Part model, mm, in its own coordinate system. Coordinates: 2 decimals unless noted, no trailing zeros. Loops run counter-clockwise (first coordinate to the right, second up) from the corner with the lowest first, then second, coordinate; pieces in that order, holes last. Notation, with made-up numbers: (84.25, 6) - (102.25, 6) arc R17 cw to (102.25, 29) - close; hole circle Ø5 at (88, 44.25). An arc over 180 degrees is marked (long way). Answer as CSV lines item,"result".
from build123d import *

# Parameters (mm, degrees)
F1_DEPTH = 1622.425
F3_DEPTH = 38.1
F5_DEPTH = 25.4


with BuildPart() as f1:
    # F0 (on Front) → F1 (new body)
    with BuildSketch(Plane.XZ):
        with BuildLine():
            Line((-10.2273916114, -12.0247762322), (8.8226083886, -12.0247762322))
            ThreePointArc((8.8226083886, -12.0247762322), (11.0676724189, -11.0948402625), (11.9976083886, -8.8497762322))
            Line((11.9976083886, -8.8497762322), (11.9976083886, 10.2002237678))
            ThreePointArc((11.9976083886, 10.2002237678), (11.0676724189, 12.445287798), (8.8226083886, 13.3752237678))
            Line((8.8226083886, 13.3752237678), (-10.2273916114, 13.3752237678))
            ThreePointArc((-10.2273916114, 13.3752237678), (-12.4724556417, 12.445287798), (-13.4023916114, 10.2002237678))
            Line((-13.4023916114, 10.2002237678), (-13.4023916114, -8.8497762322))
            ThreePointArc((-13.4023916114, -8.8497762322), (-12.4724556417, -11.0948402625), (-10.2273916114, -12.0247762322))
        make_face()
        with BuildLine():
            ThreePointArc((8.8226083886, -5.6747762322), (7.8926724189, -7.9198402625), (5.6476083886, -8.8497762322))
            Line((5.6476083886, -8.8497762322), (-7.0523916114, -8.8497762322))
            ThreePointArc((-7.0523916114, -8.8497762322), (-9.2974556417, -7.9198402625), (-10.2273916114, -5.6747762322))
            Line((-10.2273916114, -5.6747762322), (-10.2273916114, 7.0252237678))
            ThreePointArc((-10.2273916114, 7.0252237678), (-9.2974556417, 9.270287798), (-7.0523916114, 10.2002237678))
            Line((-7.0523916114, 10.2002237678), (5.6476083886, 10.2002237678))
            ThreePointArc((5.6476083886, 10.2002237678), (7.8926724189, 9.270287798), (8.8226083886, 7.0252237678))
            Line((8.8226083886, 7.0252237678), (8.8226083886, -5.6747762322))
        make_face(mode=Mode.SUBTRACT)
    extrude(amount=F1_DEPTH)

    # F2 (on Right) → F3 (cut, symmetric)
    with BuildSketch(Plane.YZ):
        Polygon((0, -13.513528793), (0, 13.375182943), (-12.9695749158, -13.513528793), align=None)
    extrude(amount=F3_DEPTH, both=True, mode=Mode.SUBTRACT)

    # F4 (on Right) → F5 (cut, symmetric)
    with BuildSketch(Plane.YZ):
        Polygon((-1622.425, 14.8639355038), (-1622.425, -12.0247762322), (-1609.4554250842, 14.8639355038), align=None)
    extrude(amount=F5_DEPTH, both=True, mode=Mode.SUBTRACT)


solid = f1.part
Q1. Saw through at A-A (y = -1335). Give the cut face in (x, z) (3 decimals), then the cut area to 3 significant figures.
Results:
outline,"(-13.402, -8.85) arc R3.175 ccw to (-10.227, -12.025) - (8.823, -12.025) arc R3.175 ccw to (11.998, -8.85) - (11.998, 10.2) arc R3.175 ccw to (8.823, 13.375) - (-10.227, 13.375) arc R3.175 ccw to (-13.402, 10.2) - close; hole (-10.227, -5.675) arc R3.175 ccw to (-7.052, -8.85) - (5.648, -8.85) arc R3.175 ccw to (8.823, -5.675) - (8.823, 7.025) arc R3.175 ccw to (5.648, 10.2) - (-7.052, 10.2) arc R3.175 ccw to (-10.227, 7.025) - close"
area,"282 mm^2"
Q2. Wall check: L1, parallel to Z at x = -9.75, y = -1484; L2, parallel to X at y = -1322, z = 4.75; L3, parallel to Z at x = 6.25, y = -1034.5. Give the ranges that are in metal, low to high.
Results:
L1,"z = -12.02 to -7.35, 8.7 to 13.38"
L2,"x = -13.4 to -10.23, 8.82 to 12"
L3,"z = -12.02 to -8.79, 10.14 to 13.38"
Q3. Flat gauge pins, fed straight in: pin 1 (3 mm diameter, centred on x = -10.5, z = -2.5, fed in from +Y); pin 2 (3 mm diameter, centred on y = -782.5, z = -9, fed in from -X); pin 3 (4 mm diameter, centred on x = 3, z = 9.5, fed in from -Y). Where does each tip first touch, or does it go through?
Results:
pin 1,"stops at y = -6.93"
pin 2,"stops at x = -13.4"
pin 3,"stops at y = -1611.7"
Q4. Saw through at B-B (z = 1). Give the cut face in (x, y).
Results:
outline,"(-13.4, -1616.14) - (-10.23, -1616.14) - (-10.23, -5.97) - (-13.4, -5.97) - close; (8.82, -1616.14) - (12, -1616.14) - (12, -5.97) - (8.82, -5.97) - close"
